```python
from build123d import *

# Parameters (mm, degrees)
SZKIC1_W                    = 596
SZKIC1_H                    = 62
DODANIE_WYCI_GNI_CIE1_DEPTH = 76
SZKIC2_R                    = 21
WYTNIJ_WYCI_GNI_CIE1_DEPTH  = 76
SZKIC3_R                    = 21
WYTNIJ_WYCI_GNI_CIE2_DEPTH  = 76
SZKIC4_W                    = 76
SZKIC4_H                    = 9
SZKIC5_W                    = 76
SZKIC5_H                    = 9


with BuildPart() as part:
    # Szkic1 → Dodanie-wyci_gni_cie1 (new body)
    with BuildSketch(Plane.XY):
        with Locations((0, 167)):
            Rectangle(SZKIC1_W, SZKIC1_H)
    extrude(amount=DODANIE_WYCI_GNI_CIE1_DEPTH)

    # Szkic2 → Wytnij-wyci_gni_cie1 (cut)
    with BuildSketch(Plane.XY.offset(76)):
        with Locations((262, 162)):
            Circle(SZKIC2_R)
    extrude(amount=-WYTNIJ_WYCI_GNI_CIE1_DEPTH, mode=Mode.SUBTRACT)

    # Szkic3 → Wytnij-wyci_gni_cie2 (cut)
    with BuildSketch(Plane.XY.offset(76)):
        with Locations((-262, 162)):
            Circle(SZKIC3_R)
    extrude(amount=-WYTNIJ_WYCI_GNI_CIE2_DEPTH, mode=Mode.SUBTRACT)

    # Szkic4 → Wyci_cie-obr_t1 (revolve, cut)
    with BuildSketch(Plane(origin=(215, 0, 0), x_dir=(0, 0, -1), z_dir=(1, 0, 0)), mode=Mode.PRIVATE) as wyci_cie_obr_t1_sk:
        with Locations((-38, 166.5)):
            Rectangle(SZKIC4_W, SZKIC4_H)
    revolve(wyci_cie_obr_t1_sk.sketch.rotate(Axis((215, 162, 0), (0, 0, 1)), 270), axis=Axis((215, 162, 0), (0, 0, 1)), mode=Mode.SUBTRACT)

    # Szkic5 → Wyci_cie-obr_t2 (revolve, cut)
    with BuildSketch(Plane(origin=(-215, 0, 0), x_dir=(0, 0, -1), z_dir=(1, 0, 0)), mode=Mode.PRIVATE) as wyci_cie_obr_t2_sk:
        with Locations((-38, 166.5)):
            Rectangle(SZKIC5_W, SZKIC5_H)
    revolve(wyci_cie_obr_t2_sk.sketch.rotate(Axis((-215, 162, 0), (0, 0, 1)), 270), axis=Axis((-215, 162, 0), (0, 0, 1)), mode=Mode.SUBTRACT)


solid = part.part
```
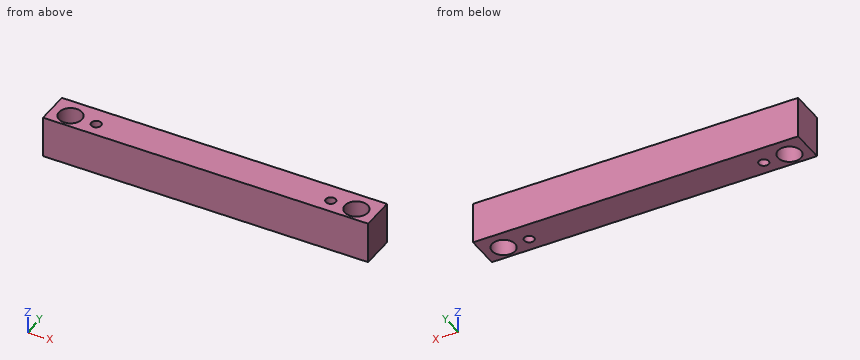
Verification items for the finished model (mm, model axes). Coordinates: 2 decimals unless noted, no trailing zeros. Loops run counter-clockwise (first coordinate to the right, second up) from the corner with the lowest first, then second, coordinate; pieces in that order, holes last. Notation, with made-up numbers: (36.5, 71.25) -> (91.5, 71.25) arc R22 cw to (91.5, 89.25) -> close; hole circle Ø5 at (-12, 60.25). An arc over 180 degrees is marked (long way). Answer in a Markdown table with one row per item. Add a question column.
1. Section check C-C, the plane z = 34. Enter the section's corners in (x, y).
2. Section check D-D, the plane x = 262. Enter the section's corners in (y, z).
3. Material ranges on probe 1 along X at (y, z) = (160, 65.5); probe 2 along Y at (x, z) = (215, 55); probe 3 along X at (y, z) = (150.5, 61.5), recorded low to high. Write a range as [from, to].
4. Section check B-B, the plane x = -215. Enter the section's corners in (y, z).
5. Section check A-A, the plane y = 162. Enter the section's corners in (x, z).
Derived:
| question | item | result |
|---|---|---|
| 1 | outline | (-298, 136) -> (298, 136) -> (298, 198) -> (-298, 198) -> close; hole circle Ø42 at (-262, 162); hole circle Ø18 at (-215, 162); hole circle Ø18 at (215, 162); hole circle Ø42 at (262, 162) |
| 2 | outline | (136, 0) -> (141, 0) -> (141, 76) -> (136, 76) -> close; (183, 0) -> (198, 0) -> (198, 76) -> (183, 76) -> close |
| 3 | probe 1 | x = [-298, -282.9], [-241.1, -223.77], [-206.23, 206.23], [223.77, 241.1], [282.9, 298] |
| 3 | probe 2 | y = [136, 153], [171, 198] |
| 3 | probe 3 | x = [-298, -279.57], [-244.43, 244.43], [279.57, 298] |
| 4 | outline | (136, 0) -> (153, 0) -> (153, 76) -> (136, 76) -> close; (171, 0) -> (198, 0) -> (198, 76) -> (171, 76) -> close |
| 5 | outline | (-298, 0) -> (-283, 0) -> (-283, 76) -> (-298, 76) -> close; (-241, 0) -> (-224, 0) -> (-224, 76) -> (-241, 76) -> close; (-206, 0) -> (206, 0) -> (206, 76) -> (-206, 76) -> close; (224, 0) -> (241, 0) -> (241, 76) -> (224, 76) -> close; (283, 0) -> (298, 0) -> (298, 76) -> (283, 76) -> close |
